Work out the finished part from the listing and answer in its coordinate system (mm). A direction names the side the tool comes from. Give positions to 0.01 mm unless a question says otherwise; leave off trailing zeros. Order: outer loops, then holes, each group sorted by start corner. A loop starts at its lowest first (then second) coordinate and runs counter-clockwise, first axis right, second up. Notation, with made-up numbers: (45.25, 48.25) - (63.25, 48.25) arc R28 ccw to (63.25, 83.25) - close; hole circle Ø6 at (-8, 31). An arc over 180 degrees is marked (long way). Write each question's results on one line, items separated by ' | '.
from build123d import *

# Parameters (mm, degrees)
F3_DEPTH  = 0.25
F4_DEPTH  = 0.25
F5_W      = 80.37
F5_H      = 7.7
F6_DEPTH  = 0.25
F8_DEPTH  = 80.37
F10_DEPTH = 80.37
F12_DEPTH = 8.2010001
F13_R     = 0.825
F14_DEPTH = 2


with BuildPart() as f3:
    # F0 (on Front) → F3 (new body)
    with BuildSketch(Plane.XZ):
        with BuildLine():
            Line((-40.185, 0.25), (-40.185, 0))
            Line((-40.185, 0), (-21.105, 0))
            Line((-21.105, 0), (-21.105, 2.7953359774))
            ThreePointArc((-21.105, 2.7953359774), (-20.2003359774, 3.7), (-19.2956719548, 2.7953359774))
            Line((-19.2956719548, 2.7953359774), (-19.2956719548, 1.3671361376))
            Line((-19.2956719548, 1.3671361376), (-15.7349420673, 1.3671361376))
            ThreePointArc((-15.7349420673, 1.3671361376), (-15.5016377941, 1.2704983434), (-15.405, 1.0371940702))
            Line((-15.405, 1.0371940702), (-15.405, 0))
            Line((-15.405, 0), (3.495, 0))
            Line((3.495, 0), (3.495, 2.98))
            Line((3.495, 2.98), (9.395, 2.98))
            Line((9.395, 2.98), (9.395, 0))
            Line((9.395, 0), (40.185, 0))
            Line((40.185, 0), (41.255, 5))
            Line((41.255, 5), (29.705, 5))
            Line((29.705, 5), (29.705, 3.55))
            Line((29.705, 3.55), (24.125, 3.55))
            Line((24.125, 3.55), (24.125, 5))
            Line((24.125, 5), (-35.445, 5))
            Line((-35.445, 5), (-43.265, 7.26))
            Line((-43.265, 7.26), (-47.025, 7.26))
            ThreePointArc((-47.025, 7.26), (-48.675, 4.76), (-50.325, 7.26))
            Line((-50.325, 7.26), (-51.985, 7.26))
            Line((-51.985, 7.26), (-51.985, 6.2604746746))
            add(Edge.make_bspline(
                [(-51.985, 6.2604746746), (-51.8611107918, 4.7384496413), (-51.1533093269, 4.1423325476), (-50.6568033495, 3.9383888915)],
                knots=[0.5835535338, 0.5835535338, 0.5835535338, 0.5835535338, 3.577318367, 3.577318367, 3.577318367, 3.577318367], degree=3))
            Line((-50.6568033495, 3.9383888915), (-40.185, 0.25))
        make_face()
    extrude(amount=F3_DEPTH)



with BuildPart() as f4:
    # F2 (on offset) → F4 (new body)
    with BuildSketch(Plane.XZ.offset(-7.7)):
        with BuildLine():
            Line((3.495, 2.98), (9.395, 2.98))
            Line((9.395, 2.98), (9.395, 0))
            Line((9.395, 0), (40.185, 0))
            Line((40.185, 0), (41.255, 5))
            Line((41.255, 5), (29.705, 5))
            Line((29.705, 5), (29.705, 3.55))
            Line((29.705, 3.55), (24.125, 3.55))
            Line((24.125, 3.55), (24.125, 5))
            Line((24.125, 5), (-35.445, 5))
            Line((-35.445, 5), (-43.265, 7.26))
            Line((-43.265, 7.26), (-47.025, 7.26))
            ThreePointArc((-47.025, 7.26), (-48.675, 4.76), (-50.325, 7.26))
            Line((-50.325, 7.26), (-51.985, 7.26))
            Line((-51.985, 7.26), (-51.985, 6.2604746746))
            add(Edge.make_bspline(
                [(-51.985, 6.2604746746), (-51.8611107918, 4.7384496413), (-51.1533093269, 4.1423325476), (-50.6568033495, 3.9383888915)],
                knots=[0.1631259715, 0.1631259715, 0.1631259715, 0.1631259715, 1, 1, 1, 1], degree=3))
            Line((-50.6568033495, 3.9383888915), (-40.185, 0.25))
            Line((-40.185, 0.25), (-40.185, 0))
            Line((-40.185, 0), (-21.105, 0))
            Line((-21.105, 0), (-15.405, 0))
            Line((-15.405, 0), (3.495, 0))
            Line((3.495, 0), (3.495, 2.98))
        make_face()
    extrude(amount=-F4_DEPTH)


with BuildPart() as f6:
    # F5 (on Top) → F6 (new body)
    with BuildSketch(Plane.XY):
        with Locations((0, 3.85)):
            Rectangle(F5_W, F5_H)
    extrude(amount=-F6_DEPTH)


with BuildPart() as f3_1:
    add(f3.part)

    add(f6.part)  # F8 merges F6
    # F7 (on face) → F8 (join, through all)
    with BuildSketch(Plane(origin=(-40.185, 0, 0), x_dir=(0, -1, 0), z_dir=(-1, 0, 0))):
        with BuildLine():
            Line((0, 0), (0, -0.25))
            ThreePointArc((0, -0.25), (0.1767766953, -0.1767766953), (0.25, 0))
            Line((0.25, 0), (0, 0))
        make_face()
    extrude(amount=-F8_DEPTH)


    add(f4.part)  # F10 merges F4
    # F9 (on face) → F10 (join, through all)
    with BuildSketch(Plane(origin=(-40.185, 0, 0), x_dir=(0, -1, 0), z_dir=(-1, 0, 0))):
        with BuildLine():
            Line((-7.7, 0), (-7.95, 0))
            ThreePointArc((-7.95, 0), (-7.8767766953, -0.1767766953), (-7.7, -0.25))
            Line((-7.7, -0.25), (-7.7, 0))
        make_face()
    extrude(amount=-F10_DEPTH)

    # F11 (on face) → F12 (cut, through all)
    with BuildSketch(Plane.XZ.offset(0.25)):
        with BuildLine():
            ThreePointArc((38.2632873952, 2.2013515081), (38.8466504897, 2.4429884136), (39.0882873952, 3.0263515081))
            ThreePointArc((39.0882873952, 3.0263515081), (38.8466504897, 3.6097146026), (38.2632873952, 3.8513515081))
            Line((38.2632873952, 3.8513515081), (38.2632873952, 2.2013515081))
        make_face()
        with BuildLine():
            Line((38.2632873952, 2.2013515081), (38.2632873952, 3.8513515081))
            ThreePointArc((38.2632873952, 3.8513515081), (37.4382873952, 3.0263515081), (38.2632873952, 2.2013515081))
        make_face()
    extrude(amount=-F12_DEPTH, mode=Mode.SUBTRACT)

    # F13 (on face) → F14 (cut)
    with BuildSketch(Plane(origin=(0, 7.95, 0), x_dir=(-1, 0, 0), z_dir=(0, 1, 0))):
        with Locations((15.0666469708, 2.5)):
            Circle(F13_R)
    extrude(amount=-F14_DEPTH, mode=Mode.SUBTRACT)


solid = f3_1.part
1. A cutting plane is placed at B-B, the plane y = 3.25. Write down the section's boundary in (x, z) (3 decimals), then the cut area to 3 significant figures.
Answer list:
outline: (-40.185, -0.25) - (40.185, -0.25) - (40.185, 0) - (-40.185, 0) - close | area: 20.1 mm^2
2. A tool of negligible diameter and unlimited length cuts with its end or side. For faces 1 (the face through (-6, -0.25, 3)), 2 (the face through (-6, 0, 3)), from which of +Z, -Z, +X, -X, +Y, -Y can it reach the whole face along a straight path? Write none if from no direction.
Answer list:
face 1: +Z, -Z, +X, -X, -Y | face 2: +Z, +X, -X
3. Straight lines are drawn through the part: line 1 (Y direction, x = -23, z = 4.5); line 2 (Z direction, x = -11, y = 7). For each, find the intervals that lie inside material, in ascending order. Write a range as [from, to].
Answer list:
line 1: [-0.25, 0], [7.7, 7.95] | line 2: [-0.25, 0]
4. A cutting plane is placed at A-A, the plane x = -2. Write down the section's boundary in (y, z), then the cut area to 3 significant figures.
Answer list:
outline: (-0.25, 0) arc R0.25 ccw to (0, -0.25) - (7.7, -0.25) arc R0.25 ccw to (7.95, 0) - (7.95, 5) - (7.7, 5) - (7.7, 0) - (0, 0) - (0, 5) - (-0.25, 5) - close | area: 4.52 mm^2
5. Given P1, Ø1, axis at y = 6, z = 4, coming from the +X side, flat-ended and moving along its own axis, determine where the tip first touches the part or whether it passes through.
Answer list:
P1: through
